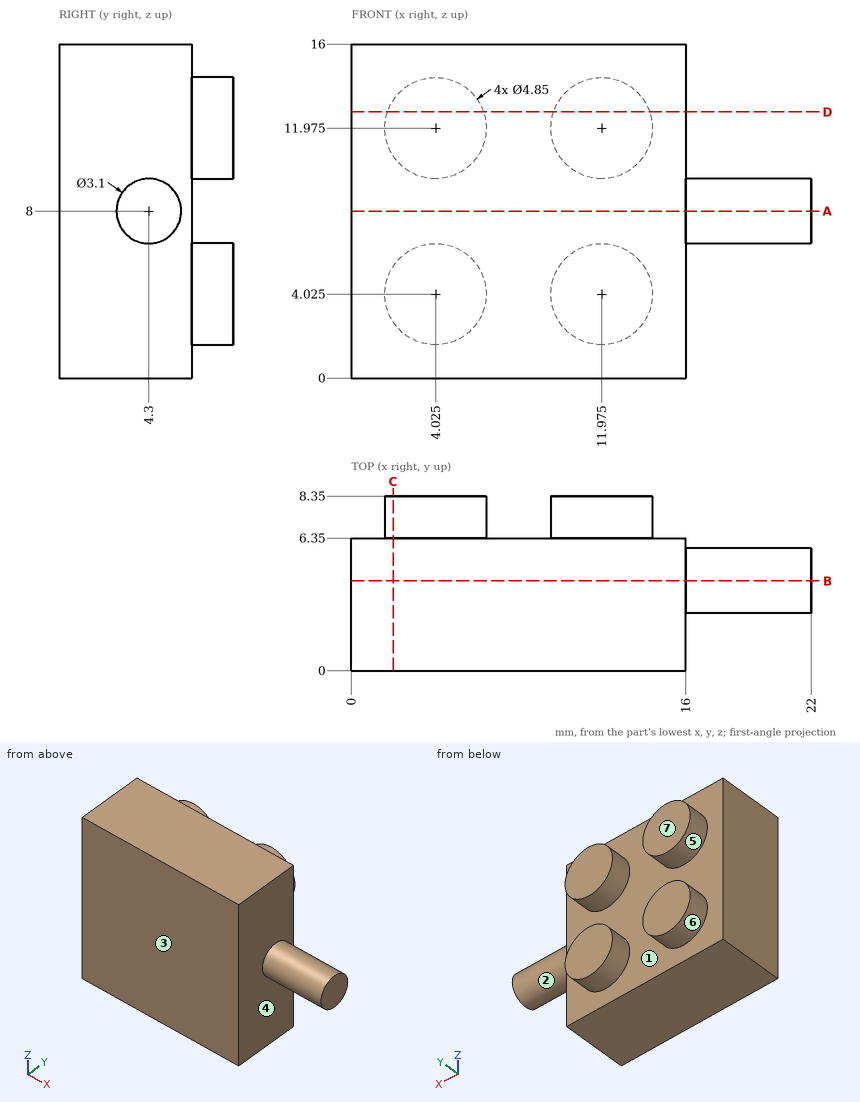
The drawing under review shows one solid part. Ordinate dimensions are in mm from its lowest x, y, z. A direction names the side the tool comes from. Coordinates: 2 decimals unless noted, no trailing zeros. Write each loop counter-clockwise with the first axis right and the second up, starting at its lowest first coordinate (ties: lowest second). Pieces come first, ordered by that corner, then holes. Notation, with made-up numbers: (30, 78) -> (66, 78) arc R18 ccw to (66, 88) -> close; hole circle Ø7 at (-32.75, -21.75). An arc over 180 degrees is marked (long way). One line per item, written item: value. Start each with the question number.
Q1. Clearance check with flat-ended pins moving along their axes: P1, Ø5, axis at x = 20, y = 5.5, coming from the +Z side; P2, Ø2, axis at y = 4.5, z = 3.5, coming from the +X side. State where each tip first meets the part, or that it passes through.
Q2. Add section C-C, the plane x = 2. Give the boundary of the cut face in (y, z).
Q3. The part is to be moulded in two halves that separate along X. For the marked faces 4, 5, 6 and 7, say which applies: +X half, -X half, draft (parallel to the pull), parting line (faces both ways), or undercut.
Q4. For the marked faces 1, 2 and 3, list the 3-axis set-ups (+Z, -Z, +X, -X, +Y, -Y) from which the entire face can be reached by the end or side of a thin tool; tool diameter is ignored.
Q5. To check wall thickness, follow probe 1 along X at (y, z) = (1, 12.5); probe 2 along Y at (x, z) = (14, 5.75); probe 3 along X at (y, z) = (7.5, 12.25). State the ranges of each line that lie inside material, in increasing order.
Q6. Add section D-D, the plane z = 12.75. Give the boundary of the cut face in (x, y), then the cut area to 3 significant figures.
Q7. Add section B-B, the plane y = 4.3. Give the boundary of the cut face in (x, z), then the cut area to 3 significant figures.
Q8. Add section A-A, the plane z = 8. Give the boundary of the cut face in (x, y), then the cut area to 3 significant figures.
Response:
1. P1: z = 9.55
1. P2: x = 16
2. outline: (0, 0) -> (6.35, 0) -> (6.35, 2.69) -> (8.35, 2.69) -> (8.35, 5.36) -> (6.35, 5.36) -> (6.35, 10.64) -> (8.35, 10.64) -> (8.35, 13.31) -> (6.35, 13.31) -> (6.35, 16) -> (0, 16) -> close
3. face 4: +X half
3. face 5: undercut
3. face 6: undercut
3. face 7: draft
4. face 1: +Y
4. face 2: +X
4. face 3: +Z, -Z, +X, -X, -Y
5. probe 1: 0 to 16
5. probe 2: 0 to 6.35
5. probe 3: 1.62 to 6.43, 9.57 to 14.38
6. outline: (0, 0) -> (16, 0) -> (16, 6.35) -> (14.27, 6.35) -> (14.27, 8.35) -> (9.68, 8.35) -> (9.68, 6.35) -> (6.32, 6.35) -> (6.32, 8.35) -> (1.73, 8.35) -> (1.73, 6.35) -> (0, 6.35) -> close
6. area: 120 mm²
7. outline: (0, 0) -> (16, 0) -> (16, 6.45) -> (22, 6.45) -> (22, 9.55) -> (16, 9.55) -> (16, 16) -> (0, 16) -> close
7. area: 275 mm²
8. outline: (0, 0) -> (16, 0) -> (16, 2.75) -> (22, 2.75) -> (22, 5.85) -> (16, 5.85) -> (16, 6.35) -> (0, 6.35) -> close
8. area: 120 mm²
